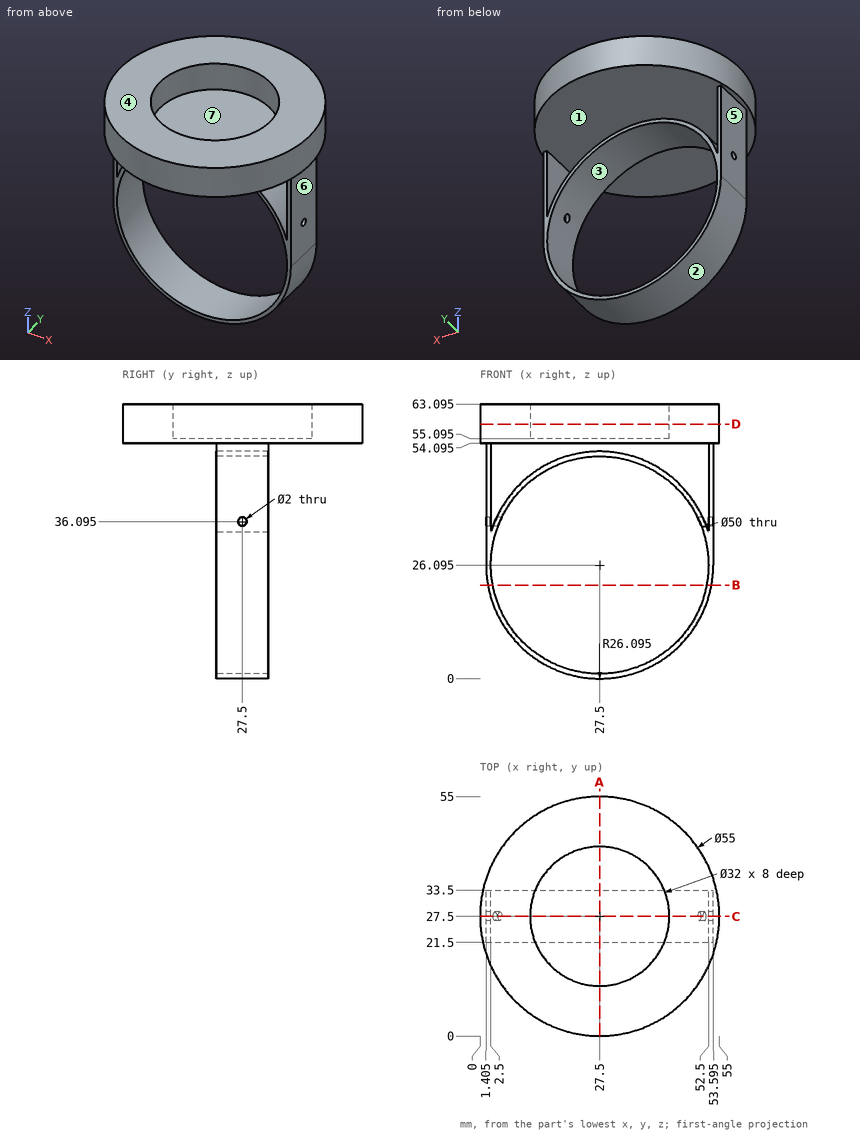
Geometry: see drawing. Coordinates: mm, zero at the bounding-box minimum. A direction names the side the tool comes from. Round coordinates to 2 decimals unless told otherwise and drop trailing zeros. Write each loop counter-clockwise with the first axis right and the second up, starting at its lowest first coordinate (ties: lowest second). Pieces come first, ordered by that corner, then holes. Notation, with made-up numbers: M 84,-6 L 118,-6 A24 cw 118,33 Z; hole C 51,-26.5 d9. An arc over 180 degrees is marked long. Answer in a Markdown table with one row per item. Add a question column.
(1) Draft query along Z for the marked faces 1, 2, 3 and 4. Return one class per face: pulls with the +Z half, pulls with the -Z half, needs draft (parallel to the pull), parting line crosses it, or undercut.
(2) Reachability of the marked faces 5, 6 and 7 from +Z, -Z, +X, -X, +Y, -Y: full face, straight path, thin tool, end or side. Return the list, or none.
(3) Cut plane C-C, the plane y = 27.5. Give the number of separate pieces and of enclosed holes in the cut face, then the cut area to 3 significant figures.
(4) Contact query for flat-ended pins moving along their axis: pin 1 (9.5 mm diameter, centred on y = 26.5, z = 47, fed in from -X) (3 decimals); pin 2 (1 mm diameter, centred on x = 12, y = 25.5, fed in from +Z) (3 decimals); pin 3 (3 mm diameter, centred on x = 49, z = 37, fed in from +Y); pin 4 (12 mm diameter, centred on x = 31, y = 34.5, fed in from +Z) (3 decimals). Output: stop coordinate, or through.
(5) Cut plane B-B, the plane z = 21.5. Return the cut outline in (x, y).
(6) Ray query, L1, parallel to Z at x = 35.5, y = 26 (1 decimal); L2, parallel to Z at x = 8, y = 39 (1 decimal); L3, parallel to X at y = 17, z = 60.5. Return the intervals inside material, ascending.
(7) Cut plane A-A, the plane x = 27.5. Return the cut outline in (y, z) (1 decimal).
(8) Cut plane D-D, the plane z = 58.5. Return the cut outline in (x, y), then the cut area to 3 significant figures.
Established:
| question | item | result |
|---|---|---|
| 1 | face 1 | undercut |
| 1 | face 2 | pulls with the -Z half |
| 1 | face 3 | undercut |
| 1 | face 4 | pulls with the +Z half |
| 2 | face 5 | -Z, -X, +Y, -Y |
| 2 | face 6 | -Z, +X, +Y, -Y |
| 2 | face 7 | +Z |
| 3 | separate pieces | 3 |
| 3 | enclosed holes | 0 |
| 3 | area | 456 mm² |
| 4 | pin 1 | x = 1.405 |
| 4 | pin 2 | z = 63.095 |
| 4 | pin 3 | y = 33.5 |
| 4 | pin 4 | z = 55.095 |
| 5 | outline | M 1.81,21.5 L 2.93,21.5 L 2.93,33.5 L 1.81,33.5 Z; M 52.07,21.5 L 53.19,21.5 L 53.19,33.5 L 52.07,33.5 Z |
| 6 | L1 | 1.3 to 2.4, 49.8 to 50.9, 54.1 to 55.1 |
| 6 | L2 | 54.1 to 63.1 |
| 6 | L3 | 2.08 to 15.43, 39.57 to 52.92 |
| 7 | outline | M 0,54.1 L 55,54.1 L 55,63.1 L 43.5,63.1 L 43.5,55.1 L 11.5,55.1 L 11.5,63.1 L 0,63.1 Z; M 21.5,0 L 33.5,0 L 33.5,1.1 L 21.5,1.1 Z; M 21.5,51.1 L 33.5,51.1 L 33.5,52.2 L 21.5,52.2 Z |
| 8 | outline | C 27.5,27.5 d55; hole C 27.5,27.5 d32 |
| 8 | area | 1,570 mm² |
